Model file for the job. Use its own axes, mm. Round coordinates to 2 decimals unless told otherwise and drop trailing zeros. Order: outer loops, then holes, each group sorted by start corner. A loop starts at its lowest first (then second) coordinate and runs counter-clockwise, first axis right, second up. Notation, with made-up numbers: M 89,-26.5 L 148,-26.5 A21 ccw 148,-12.5 Z; hole C -10.75,32 d5. An arc over 180 degrees is marked long. Return JSON: item names as keys, results as strings. Group by question number.
Item 1: Probe line 1 along Y through (x, z) = (0, -0.15); line 2 along X through (y, z) = (-2.5, -0.2); line 3 along Y through (x, z) = (9, 0.3). List the from-to ranges inside material, lowest first.
Item 2: Slice it at C-C on z = 0. Write the cut outline in (x, y).
Item 3: Pull direction X, two halves, no side cores. Call faces 1 (the face through (9.139, 14.334, 0.006)), 2 (the face through (7.768, 12.184, -0.006)), 3 (the face through (7, 13, -0.5)): pulls with the +X half, pulls with the -X half, needs draft (parallel to the pull), parting line crosses it, or undercut.
Item 4: Slice it at A-A on y = 0. Write the cut outline in (x, z).
from build123d import *

# Parameters (mm, degrees)
F0_R     = 17
F0_R_2   = 16
F0_R_3   = 14.45
F1_DEPTH = 0.5
F2_SIZE  = 0.1
F4_SIZE  = 0.1


with BuildPart() as f1:
    # F0 (on Top) → F1 (new body, symmetric)
    with BuildSketch(Plane.XY):
        Circle(F0_R)
        Circle(F0_R_2, mode=Mode.SUBTRACT)
        Circle(F0_R_2)
        Circle(F0_R_3, mode=Mode.SUBTRACT)
    extrude(amount=F1_DEPTH, both=True)

    # F2
    f2_edges = [f1.edges().sort_by_distance(p)[0] for p in [
        (-17, 0, 0.5),
        (-17, 0, -0.5),
    ]]
    chamfer(f2_edges, length=F2_SIZE)

    # F4
    f4_edges = [f1.edges().sort_by_distance(p)[0] for p in [
        (-14.45, 0, 0.5),
        (-14.45, 0, -0.5),
    ]]
    chamfer(f4_edges, length=F4_SIZE)


solid = f1.part
Output values:
{
 "1": {"line 1": "-17 to -14.45, 14.45 to 17", "line 2": "-16.82 to -14.23, 14.23 to 16.82", "line 3": "-14.42 to -11.3, 11.3 to 14.42"},
 "2": {"outline": "C 0,0 d34; hole C 0,0 d28.9"},
 "3": {"face 1": "parting line crosses it", "face 2": "undercut", "face 3": "needs draft"},
 "4": {"outline": "M -17,-0.4 L -16.9,-0.5 L -14.55,-0.5 L -14.45,-0.4 L -14.45,0.4 L -14.55,0.5 L -16.9,0.5 L -17,0.4 Z; M 14.45,-0.4 L 14.55,-0.5 L 16.9,-0.5 L 17,-0.4 L 17,0.4 L 16.9,0.5 L 14.55,0.5 L 14.45,0.4 Z"}
}
